Check sheet for the drawn part. Datum: minimum x, y, z corner. Units: mm. A direction names the side the tool comes from. Coordinates: 2 decimals unless noted, no trailing zeros. Write each loop counter-clockwise with the first axis right and the second up, starting at its lowest first coordinate (ties: lowest second). Pieces come first, ordered by that corner, then holes. Notation, with made-up numbers: (49.5, 46.25) -> (98.5, 46.25) arc R27 cw to (98.5, 65.25) -> close; hole circle Ø3 at (-40, -16). An arc over 180 degrees is marked (long way). Answer in a Markdown table with one row per item. Add a question column.
Q1. Release check for a two-part mould opening along Y. For the marked faces 5, 6 and 7 record: pulls with the +Y half, pulls with the -Y half, needs draft (parallel to the pull), parting line crosses it, or undercut.
Q2. Gauge pin test, flat ends, axial feed: P1, Ø15, axis at x = 78, z = 25, coming from the -Y side; P2, Ø8, axis at y = 7, z = 26.5, coming from the +X side; P3, Ø13.5, axis at x = 13.85, z = 25, coming from the -Y side; P4, Ø1.5, axis at y = 82.5, z = 40.5, coming from the -X side. Record the tip position at first contact, or that the pin passes through.
Q3. Section check D-D, the plane z = 46.5. Record the boundary of the cut face in (x, y).
Q4. Section check A-A, the plane y = 35. Record the boundary of the cut face in (x, z), and give its area (3 significant figures).
Q5. Thickness scan on line 1 (X direction, y = 18.25, z = 25); line 2 (Y direction, x = 64, z = 15.5); line 3 (Y direction, x = 40.5, z = 18). Record the ranges inside material, lowest first.
Q6. Section check C-C, the plane z = 25. Record the boundary of the cut face in (x, y), and give its area (3 significant figures).
Q7. Section check B-B, the plane x = 45. Record the boundary of the cut face in (y, z), and give its area (3 significant figures).
Q8. Tool access check on the marked faces 1, 2, 3 and 4. Record the directions out of +Z, -Z, +X, -X, +Y, -Y that give a thin tool (end or side, any length) a straight path to the whole face; none if there is none.
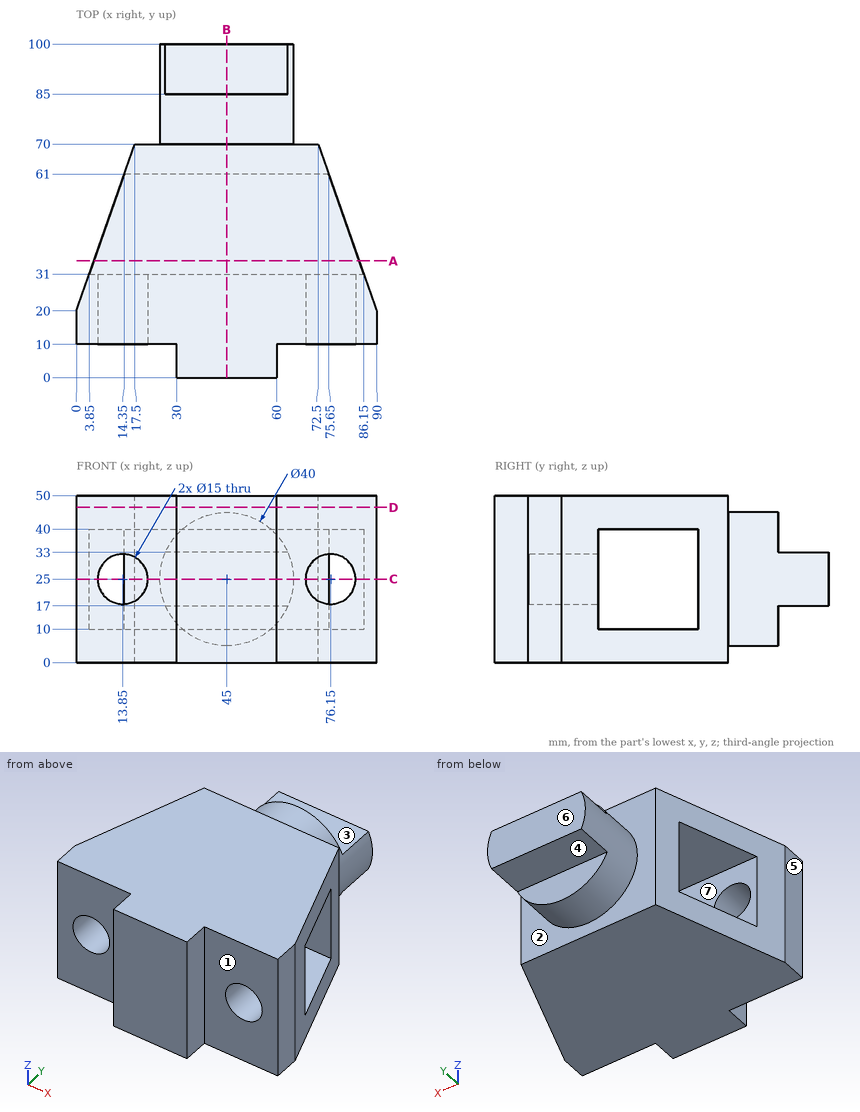
Calculated:
| question | item | result |
|---|---|---|
| 1 | face 5 | needs draft |
| 1 | face 6 | pulls with the +Y half |
| 1 | face 7 | undercut |
| 2 | P1 | stops at y = 10 |
| 2 | P2 | stops at x = 90 |
| 2 | P3 | stops at y = 61 |
| 2 | P4 | stops at x = 31.49 |
| 3 | outline | (0, 10) -> (30, 10) -> (30, 0) -> (60, 0) -> (60, 10) -> (90, 10) -> (90, 20) -> (72.5, 70) -> (17.5, 70) -> (0, 20) -> close |
| 4 | outline | (5.25, 0) -> (84.75, 0) -> (84.75, 10) -> (5.25, 10) -> close; (5.25, 40) -> (84.75, 40) -> (84.75, 50) -> (5.25, 50) -> close |
| 4 | area | 1,590 mm² |
| 5 | line 1 | x = 0 to 6.35, 21.35 to 68.65, 83.65 to 90 |
| 5 | line 2 | y = 10 to 31, 61 to 70 |
| 5 | line 3 | y = 0 to 31, 61 to 100 |
| 6 | outline | (0, 10) -> (6.35, 10) -> (6.35, 31) -> (3.85, 31) -> (0, 20) -> close; (14.35, 61) -> (75.65, 61) -> (72.5, 70) -> (65, 70) -> (65, 100) -> (25, 100) -> (25, 70) -> (17.5, 70) -> close; (21.35, 10) -> (30, 10) -> (30, 0) -> (60, 0) -> (60, 10) -> (68.65, 10) -> (68.65, 31) -> (21.35, 31) -> close; (83.65, 10) -> (90, 10) -> (90, 20) -> (86.15, 31) -> (83.65, 31) -> close |
| 6 | area | 3,240 mm² |
| 7 | outline | (0, 0) -> (70, 0) -> (70, 5) -> (85, 5) -> (85, 17) -> (100, 17) -> (100, 33) -> (85, 33) -> (85, 45) -> (70, 45) -> (70, 50) -> (0, 50) -> close; hole (31, 10) -> (61, 10) -> (61, 40) -> (31, 40) -> close |
| 7 | area | 3,440 mm² |
| 8 | face 1 | +Z, -Z, +X, -Y |
| 8 | face 2 | +Y |
| 8 | face 3 | +Z, +X, -X, +Y |
| 8 | face 4 | -Z, +X, -X, +Y |
